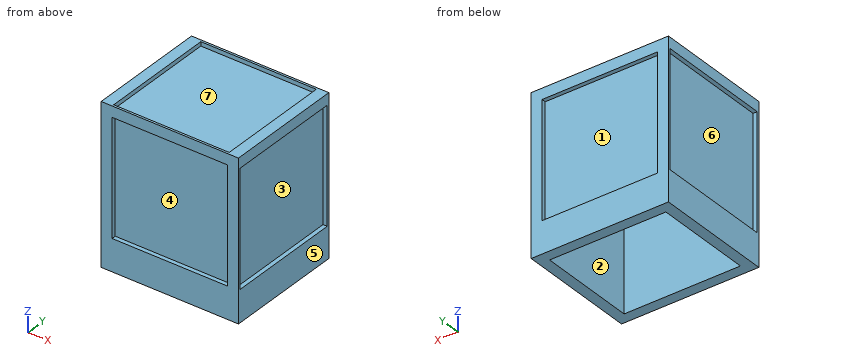
Autodesk Inventor part; units mm, degrees
ref_plane "YZ Plane" through (0, 0, 0) normal (1, 0, 0) x (0, 1, 0)
ref_plane "XZ Plane" through (0, 0, 0) normal (0, 1, 0) x (-1, 0, 0)
ref_plane "XY Plane" through (0, 0, 0) normal (0, 0, 1) x (1, 0, 0)
sketch "Sketch3" plane through (0, 0, 0) normal (0, 0, 1) x (1, 0, 0)
  line L0 (0, 0) -> (-55.38, 0)
  line L1 (-55.38, 0) -> (-55.38, 47.03)
  line L2 (-55.38, 47.03) -> (0, 47.03)
  line L3 (0, 47.03) -> (0, 0)
  line L4 (5, -5) -> (5, 52.03)
  line L5 (5, 52.03) -> (-60.38, 52.03)
  line L6 (5, -5) -> (-60.38, -5)
  line L7 (-60.38, -5) -> (-60.38, 52.03)
  dimension "d26" = 47.03
  dimension "d27" = 55.38
extrude "Extrusion10" add sketch "Sketch3" along normal blind 70.31
sketch "Sketch12" plane through (0, 0, 70.31) normal (0, 0, 1) x (1, 0, 0)
  line L0 (5, -5) -> (5, 52.03)
  line L1 (-60.38, 52.03) -> (-60.38, -5)
  line L2 (5, -5) -> (-60.38, -5)
  line L3 (-60.38, -5) -> (-60.38, 52.03)
  line L4 (-60.38, 52.03) -> (5, 52.03)
  line L5 (5, 52.03) -> (5, -5)
  point P0 (0, 0)
extrude "Extrusion13" add sketch "Sketch12" along normal blind 5
sketch "Sketch13" plane through (0, 0, 75.31) normal (0, 0, 1) x (1, 0, 0)
  line L0 (5, -5) -> (5, 52.03)
  line L1 (5, -5) -> (10.19, -5) construction
  line L2 (-60.38, -5) -> (5, -5)
  line L3 (-0.19, -5) -> (0.825, -5) construction
  line L4 (-0.19, -3.985) -> (-55.19, -3.985)
  line L5 (-55.19, -3.985) -> (-55.19, 51.015)
  line L6 (-55.19, 51.015) -> (-0.19, 51.015)
  line L7 (-0.19, 51.015) -> (-0.19, -3.985)
  point P0 (0, 0)
  dimension "d86" = 5.19
  dimension "d88" = 1.015
  dimension "d90" = 55
  dimension "d91" = 55
extrude "Extrusion14" cut sketch "Sketch13" against normal blind 2
sketch "Sketch14" plane through (-60.38, 52.03, 0) normal (0, 1, 0) x (1, 0, 0)
  line L0 (0, -75.31) -> (65.38, -75.31)
  line L1 (65.38, -75.31) -> (60.19, -75.31)
  line L2 (65.38, -75.31) -> (70.57, -75.31) construction
  line L3 (60.19, -75.31) -> (60.19, -70.155)
  line L4 (60.19, -75.31) -> (65.345, -75.31) construction
  line L5 (60.19, -70.155) -> (5.19, -70.155)
  line L6 (5.19, -70.155) -> (5.19, -15.155)
  line L7 (5.19, -15.155) -> (60.19, -15.155)
  line L8 (60.19, -15.155) -> (60.19, -70.155)
  point P0 (60.38, 0)
  dimension "d94" = 5.19
  dimension "d95" = 180
  dimension "d96" = 5.155
  dimension "d97" = 90
  dimension "d98" = 55
  dimension "d99" = 55
extrude "Extrusion15" cut sketch "Sketch14" against normal blind 2
sketch "Sketch15" plane through (-60.38, -5, 0) normal (0, -1, 0) x (1, 0, 0)
  line L0 (0, 75.31) -> (5.19, 75.31)
  line L1 (65.38, 75.31) -> (0, 75.31)
  line L2 (60.19, 70.155) -> (5.19, 70.155)
  line L3 (5.19, 75.31) -> (5.19, 70.155)
  line L4 (5.19, 70.155) -> (60.19, 70.155)
  line L5 (60.19, 70.155) -> (60.19, 15.155)
  line L6 (60.19, 15.155) -> (5.19, 15.155)
  line L7 (5.19, 15.155) -> (5.19, 70.155)
  point P0 (60.38, 0)
  point P1 (60.19, 70.155)
  dimension "d104" = 5.19
  dimension "d105" = 5.155
  dimension "d106" = 90
  dimension "d107" = 55
  dimension "d108" = 55
extrude "Extrusion16" cut sketch "Sketch15" against normal blind 2
sketch "Sketch16" plane through (-60.38, -5, 0) normal (-1, 0, 0) x (0, 0, 1)
  line L0 (0, 57.03) -> (15.155, 57.03)
  line L1 (0, 57.03) -> (15.155, 57.03) construction
  line L2 (15.155, 57.03) -> (15.155, 56.015)
  line L3 (15.155, 56.015) -> (70.155, 56.015)
  line L4 (70.155, 56.015) -> (70.155, 1.015)
  line L5 (70.155, 1.015) -> (15.155, 1.015)
  line L6 (15.155, 1.015) -> (15.155, 56.015)
  point P0 (0, 5)
  dimension "d111" = 15.155
  dimension "d112" = 0
  dimension "d113" = 1.015
  dimension "d114" = 90
  dimension "d115" = 55
  dimension "d116" = 55
extrude "Extrusion17" cut sketch "Sketch16" against normal blind 2
sketch "Sketch17" plane through (5, -5, 0) normal (1, 0, 0) x (0, 0, -1)
  line L0 (0, 57.03) -> (-75.31, 57.03)
  line L1 (-75.31, 57.03) -> (-70.155, 57.03)
  line L2 (-75.31, 57.03) -> (-70.155, 57.03) construction
  line L3 (-70.155, 57.03) -> (-70.155, 56.015)
  line L4 (-70.155, 57.03) -> (-69.14, 57.03) construction
  line L5 (-70.155, 56.015) -> (-15.155, 56.015)
  line L6 (-15.155, 56.015) -> (-15.155, 1.015)
  line L7 (-15.155, 1.015) -> (-70.155, 1.015)
  line L8 (-70.155, 1.015) -> (-70.155, 56.015)
  point P0 (0, 5)
  dimension "d119" = 5.155
  dimension "d120" = 0
  dimension "d121" = 1.015
  dimension "d122" = 90
  dimension "d123" = 55
  dimension "d124" = 55
extrude "Extrusion18" cut sketch "Sketch17" against normal blind 2
properties part number "End-Effector"
Work out the finished part from the listing and answer in its coordinate system (mm). Face numbers are marked on the shaded views. A direction names the side the tool comes from. Round coordinates to 2 decimals unless told otherwise and drop trailing zeros. Write each loop counter-clockwise with the first axis right and the second up, starting at its lowest first coordinate (ties: lowest second). Pieces come first, ordered by that corner, then holes. Notation, with made-up numbers: (-21, 35) - (27, 35) arc R27 cw to (27, 64) - close; hole circle Ø2 at (48.25, 55.25). An arc over 180 degrees is marked (long way). Return JSON: item names as keys, results as strings. Group by question number.
Q1. The mould has two halves that part along Z. Classify the marked faces 5, 6 and 7: released by +Z, released by -Z, zero draft, split by the parting line, or undercut.
Q2. The part is cut by section A-A on z = 31. Write down the section's boundary in (x, y) (3 decimals).
Q3. The part is cut by section C-C on y = 30. Write down the section's boundary in (x, z) (3 decimals), then the cut area to 3 significant figures.
Q4. The part is cut by section B-B on x = -33. Write down the section's boundary in (y, z) (3 decimals), then the cut area to 3 significant figures.
Q5. Each of these flat-tipped pins is pushed along its axis until it touches: pin 1 Ø3 at (x, z) = (-40.5, 43) entering from -Y; pin 2 Ø1.5 at (x, z) = (-1.5, 36) entering from +Y; pin 3 Ø4 at (x, y) = (-42, 38.5) entering from -Z. Where does it stop, or does it pass through?
Q6. Find the intervals of material crossed by L1, parallel to X at y = 35.5, z = 41.5; L2, parallel to Y at x = -48, z = 62.5; L3, parallel to Y at x = -40, z = 13, in increasing order.
Q7. For the marked faces 1, 2, 3 and 4, determine the directions among +Z, -Z, +X, -X, +Y, -Y from which every point of the face is accessible in a straight line to the end or side of a thin tool.
Solved:
{
 "1": {"face 5": "zero draft", "face 6": "undercut", "face 7": "released by +Z"},
 "2": {"outline": "(-60.38, -5) - (-55.19, -5) - (-55.19, -3) - (-0.19, -3) - (-0.19, -5) - (5, -5) - (5, -3.985) - (3, -3.985) - (3, 51.015) - (5, 51.015) - (5, 52.03) - (-0.19, 52.03) - (-0.19, 50.03) - (-55.19, 50.03) - (-55.19, 52.03) - (-60.38, 52.03) - (-60.38, 51.015) - (-58.38, 51.015) - (-58.38, -3.985) - (-60.38, -3.985) - close; hole (-55.38, 0) - (0, 0) - (0, 47.03) - (-55.38, 47.03) - close"},
 "3": {"outline": "(-60.38, 0) - (-55.38, 0) - (-55.38, 70.31) - (0, 70.31) - (0, 0) - (5, 0) - (5, 15.155) - (3, 15.155) - (3, 70.155) - (5, 70.155) - (5, 75.31) - (-0.19, 75.31) - (-0.19, 73.31) - (-55.19, 73.31) - (-55.19, 75.31) - (-60.38, 75.31) - (-60.38, 70.155) - (-58.38, 70.155) - (-58.38, 15.155) - (-60.38, 15.155) - close", "area": "700 mm²"},
 "4": {"outline": "(-5, 0) - (0, 0) - (0, 70.31) - (47.03, 70.31) - (47.03, 0) - (52.03, 0) - (52.03, 15.155) - (50.03, 15.155) - (50.03, 70.155) - (52.03, 70.155) - (52.03, 75.31) - (51.015, 75.31) - (51.015, 73.31) - (-3.985, 73.31) - (-3.985, 75.31) - (-5, 75.31) - (-5, 70.155) - (-3, 70.155) - (-3, 15.155) - (-5, 15.155) - close", "area": "658 mm²"},
 "5": {"pin 1": "y = -3", "pin 2": "y = 50.03", "pin 3": "z = 70.31"},
 "6": {"L1": "-58.38 to -55.38, 0 to 3", "L2": "-3 to 0, 47.03 to 50.03", "L3": "-5 to 0, 47.03 to 52.03"},
 "7": {"face 1": "+Y", "face 2": "-Z", "face 3": "+X", "face 4": "-Y"}
}
